from build123d import *

# Parameters (mm, degrees)
F1_DEPTH = 163.398445
F2_R     = 27.403209
F3_R     = 43.528601


with BuildPart() as f1:
    # F0 (on Front) → F1 (new body)
    with BuildSketch(Plane.XZ):
        Polygon((23.431614, -21.278546), (23.431614, 21.278546), (-9.84086, 47.812458), (-51.330956, 38.342614), (-69.795786, 0), (-51.330956, -38.342614), (-9.84086, -47.812458), align=None)
    extrude(amount=F1_DEPTH)

    # F2
    f2_edges = [f1.edges().sort_by_distance(p)[0] for p in [
        (-30.585908, -163.398445, 43.077536),
        (-60.563371, -163.398445, 19.171307),
        (-60.563371, -163.398445, -19.171307),
        (-30.585908, -163.398445, -43.077536),
        (6.795377, -163.398445, 34.545502),
        (23.431614, -163.398445, 0),
        (6.795377, -163.398445, -34.545502),
    ]]
    fillet(f2_edges, radius=F2_R)

    # F3
    f3_edges = [f1.edges().sort_by_distance(p)[0] for p in [
        (-30.585908, 0, 43.077536),
        (6.795377, 0, 34.545502),
        (23.431614, 0, 0),
        (6.795377, 0, -34.545502),
        (-30.585908, 0, -43.077536),
        (-60.563371, 0, 19.171307),
        (-60.563371, 0, -19.171307),
    ]]
    fillet(f3_edges, radius=F3_R)


solid = f1.part
Geometry check sheet. Reference: the model listing, model coordinates, mm. Give positions to 0.01 mm unless a question says otherwise; leave off trailing zeros. Order: outer loops, then holes, each group sorted by start corner. A loop starts at its lowest first (then second) coordinate and runs counter-clockwise, first axis right, second up. Notation, with made-up numbers: M 35.5,-34 L 40.5,-34 A35 cw 40.5,3 Z; hole C 36.25,-26 d10. An arc over 180 degrees is marked long. Use a Markdown table: item, result.
Item 1: Depth check by flat-ended pin: P1, Ø6, axis at x = -21.5, z = -13.5, coming from the +Y side; P2, Ø4, axis at y = -79.5, z = -28.5, coming from the -X side; P3, Ø1.5, axis at x = 7.5, y = -70.5, coming from the -Z side. Enter the tip coordinate at first touch or a pass-through.
Answers follow:
| item | result |
|---|---|
| P1 | stops at y = -1.09 |
| P2 | stops at x = -57.03 |
| P3 | stops at z = -34.58 |
Item 2: Section check A-A (y = -66). Record the cut outline in (x, z).
Answers follow:
| item | result |
|---|---|
| outline | M -69.8,0 L -51.33,-38.34 L -9.84,-47.81 L 23.43,-21.28 L 23.43,21.28 L -9.84,47.81 L -51.33,38.34 Z |
Item 3: Section check B-B (y = -146). Record the cut outline in (x, z).
Answers follow:
| item | result |
|---|---|
| outline | M -67.7,0 L -50.02,-36.7 L -10.31,-45.77 L 21.54,-20.37 L 21.54,20.37 L -10.31,45.77 L -50.02,36.7 Z |
Item 4: Material ranges on line 1 along X through (y, z) = (-100.5, -20.5); line 2 along Y through (x, z) = (-24.5, -36); line 3 along Z through (x, y) = (-57, -147.5), recorded low to high.
Answers follow:
| item | result |
|---|---|
| line 1 | x = -59.92 to 23.43 |
| line 2 | y = -155.6 to -18.02 |
| line 3 | z = -20.74 to 20.74 |
